Can you work these out from the drawing? Everything is in mm from the part's minimum corner. Give positions to 0.01 mm unless a question says otherwise; leave off trailing zeros. Order: outer loops, then holes, each group sorted by start corner. A loop starts at its lowest first (then second) coordinate and runs counter-clockwise, first axis right, second up. Notation, with made-up numbers: M -4,81 L 23,81 A19 cw 23,87 Z; hole C 49,29.5 d9. An arc over 180 degrees is marked long. Answer in a Markdown table with one row per item. Add a question column.
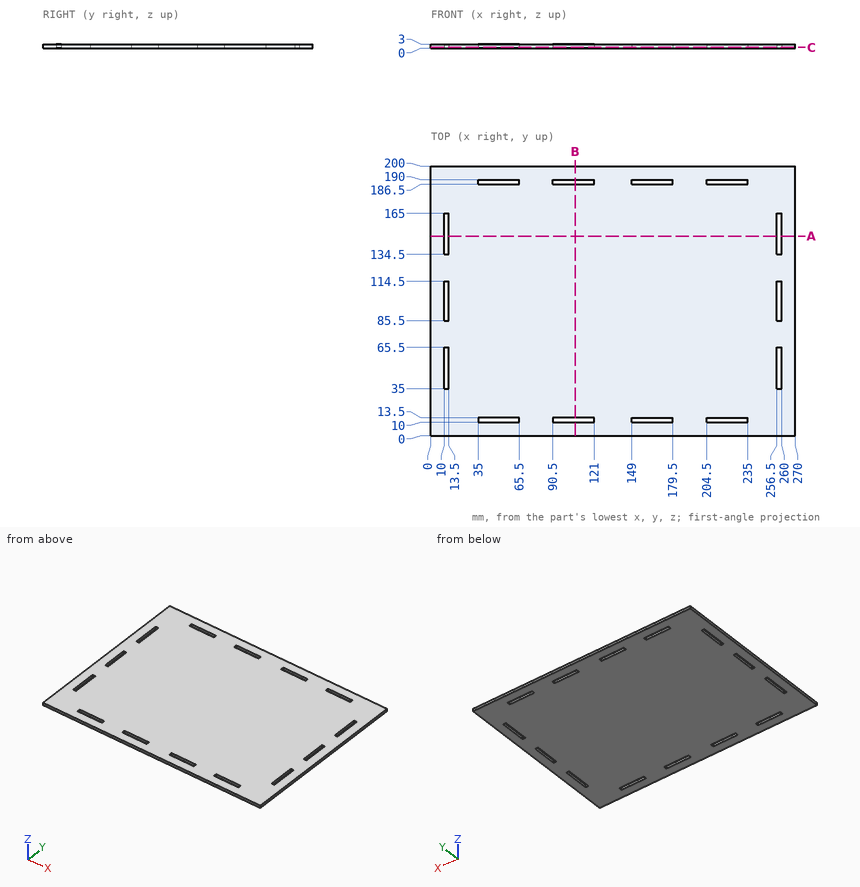
1. Suppose I cut it at C-C on z = 0.5. Count the separate pieces of the cut face and the enclosed holes in it, plus the area to 3 significant figures.
2. Suppose I cut it at A-A on y = 148. List the corners of the cut face in (x, z) for me.
3. Suppose I cut it at B-B on x = 107. List the corners of the cut face in (y, z) for me, plus the area to 3 significant figures.
4. If I drill on line 1 along Y through (x, z) = (113.5, 0.7); line 2 along Y through (x, z) = (13, 2.5); line 3 along X through (y, z) = (110.5, 1), over which ranges is the centre line in solid material (lowest first)? Write a range as [from, to].
Findings below:
| question | item | result |
|---|---|---|
| 1 | separate pieces | 1 |
| 1 | enclosed holes | 14 |
| 1 | area | 52,500 mm2 |
| 2 | outline | M 0,0 L 10,0 L 10,3 L 0,3 Z; M 13.5,0 L 256.5,0 L 256.5,3 L 13.5,3 Z; M 260,0 L 270,0 L 270,3 L 260,3 Z |
| 3 | outline | M 0,0 L 10,0 L 10,3 L 0,3 Z; M 13.5,0 L 186.5,0 L 186.5,3 L 13.5,3 Z; M 190,0 L 200,0 L 200,3 L 190,3 Z |
| 3 | area | 579 mm2 |
| 4 | line 1 | [0, 10], [13.5, 186.5], [190, 200] |
| 4 | line 2 | [0, 35], [65.5, 85.5], [114.5, 134.5], [165, 200] |
| 4 | line 3 | [0, 10], [13.5, 256.5], [260, 270] |
